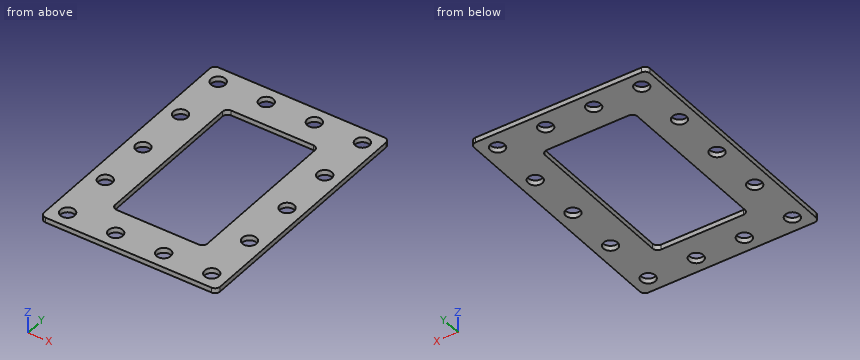
Autodesk Inventor part; units mm, degrees
ref_plane "YZ Plane" through (0, 0, 0) normal (1, 0, 0) x (0, 1, 0)
ref_plane "XZ Plane" through (0, 0, 0) normal (0, 1, 0) x (-1, 0, 0)
ref_plane "XY Plane" through (0, 0, 0) normal (0, 0, 1) x (1, 0, 0)
sketch "Sketch2" plane through (0, 0, 0) normal (0, 0, 1) x (1, 0, 0)
  line L0 (-55, -98) -> (55, -98)
  line L1 (55, -98) -> (55, 98)
  line L2 (55, 98) -> (-55, 98)
  line L3 (-55, 98) -> (-55, -98)
  line L4 (-55, -98) -> (55, 98) construction
  line L5 (55, -98) -> (-55, 98) construction
  line L6 (-105, -148) -> (105, -148)
  line L7 (105, -148) -> (105, 148)
  line L8 (105, 148) -> (-105, 148)
  line L9 (-105, 148) -> (-105, -148)
  point P0 (0, 0)
  dimension "d29" = 110
  dimension "d30" = 196
  dimension "d31" = 50
extrude "Plate2" add sketch "Sketch2" along normal blind 6
sketch "Sketch5" plane through (0, 0, 6) normal (0, 0, 1) x (1, 0, 0)
  line L0 (55, 98) -> (55, -98) construction
  line L1 (55, -98) -> (-55, -98) construction
  line L2 (-55, -98) -> (-55, 98) construction
  line L3 (-55, 98) -> (55, 98) construction
  line L4 (105, -148) -> (-105, -148) construction
  line L5 (105, 148) -> (105, -148) construction
  line L6 (-105, 148) -> (105, 148) construction
  line L7 (-105, -148) -> (-105, 148) construction
  line L8 (-86, 129) -> (86, 129) construction
  line L9 (86, 129) -> (86, -129) construction
  line L10 (86, -129) -> (-86, -129) construction
  line L11 (-86, -129) -> (-86, 129) construction
  line L12 (-55, 0) -> (55, 0) construction
  line L13 (0, 98) -> (0, -98)
  point P0 (0, 0)
  point P1 (0, -129)
  point P2 (-86, 64.5)
  point P3 (-86, 0)
  point P4 (-86, -64.5)
  point P5 (-28.6667, -129)
  point P6 (28.6667, -129)
  point P7 (86, -64.5)
  point P8 (86, 0)
  point P9 (86, 64.5)
  point P10 (28.6667, 129)
  point P11 (-28.6667, 129)
  dimension "d34" = 19
  dimension "d49" = 64.5
  dimension "d50" = 64.5
  dimension "d51" = 57.3333
  dimension "d52" = 57.3333
  dimension "d53" = 57.3333
fillet "Corner Round1" radius 6 8 edges at (-105, -148, 3) (-105, 148, 3) (105, 148, 3) (105, -148, 3) (55, -98, 3) (-55, -98, 3) (-55, 98, 3) (55, 98, 3)
hole "Hole1" at (-86, 129, 6) at (-86, 64.5, 6) at (-86, 0, 6) at (-86, -64.5, 6) at (-86, -129, 6) at (-28.6667, -129, 6) at (28.6667, -129, 6) at (86, -129, 6) at (86, -64.5, 6) at (86, 0, 6) at (86, 64.5, 6) at (86, 129, 6) at (28.6667, 129, 6) at (-28.6667, 129, 6) direction (0, 0, -1) diameter 17 end through all
equation "\"d29\" = ChargingHatch_hight - 2 * Thickness"
equation "\"d30\" = ChargingHatch_width - 2 * Thickness"
equation "\"d59\" = Thickness"
equation "\"d14\" = Thickness"
equation "\"BendReliefWidth\" = Thickness"
equation "\"BendReliefDepth\" = 0.5 * Thickness"
equation "\"CornerReliefSize\" = 4 * Thickness"
equation "\"MinimumRemnant\" = 2 * Thickness"
equation "\"TransitionRadius\" = BendRadius"
equation "\"JacobiRadiusSize\" = BendRadius"
equation "\"GapSize\" = Thickness"
properties part number "PRS 9606 charging flange round_D1200" material "Steel"
Design review of the part built by this model. Coordinates are the model's own, in mm. Coordinates: 2 decimals unless noted, no trailing zeros. Loops run counter-clockwise (first coordinate to the right, second up) from the corner with the lowest first, then second, coordinate; pieces in that order, holes last. Notation, with made-up numbers: M 76,66.25 L 120,66.25 A13 cw 120,73.25 Z; hole C 41.25,3 d8. An arc over 180 degrees is marked long. Use one line per item in the form item = value.
(1) Consider section C-C (y = -64.5). Write out the cut boundary in (x, z).
Return value:
outline = M -105,0 L -94.5,0 L -94.5,6 L -105,6 Z; M -77.5,0 L -55,0 L -55,6 L -77.5,6 Z; M 55,0 L 77.5,0 L 77.5,6 L 55,6 Z; M 94.5,0 L 105,0 L 105,6 L 94.5,6 Z
(2) Consider section A-A (y = 85). Write out the cut boundary in (x, z), and give its area (3 significant figures).
Return value:
outline = M -105,0 L -55,0 L -55,6 L -105,6 Z; M 55,0 L 105,0 L 105,6 L 55,6 Z
area = 600 mm2
(3) Clearance check with flat-ended pins moving along their axes: P1, Ø13.5, axis at x = 86, y = 129, coming from the +Z side; P2, Ø19.5, axis at x = 86, y = -64.5, coming from the -Z side. State where each tip first meets the part, or that it passes through.
Return value:
P1 = through
P2 = 0
(4) Consider section B-B (x = -86). Write out the cut boundary in (y, z), and give its area (3 significant figures).
Return value:
outline = M -148,0 L -137.5,0 L -137.5,6 L -148,6 Z; M -120.5,0 L -73,0 L -73,6 L -120.5,6 Z; M -56,0 L -8.5,0 L -8.5,6 L -56,6 Z; M 8.5,0 L 56,0 L 56,6 L 8.5,6 Z; M 73,0 L 120.5,0 L 120.5,6 L 73,6 Z; M 137.5,0 L 148,0 L 148,6 L 137.5,6 Z
area = 1,270 mm2
(5) For line 1 along X through (y, z) = (129, 3.2); line 2 along Y through (x, z) = (-86, 2.9); line 3 along X through (y, z) = (-64.5, 2), list the stretches that pass through material, from the lowest coordinate up. Write a range as from..to.
Return value:
line_1 = -105..-94.5, -77.5..-37.17, -20.17..20.17, 37.17..77.5, 94.5..105
line_2 = -148..-137.5, -120.5..-73, -56..-8.5, 8.5..56, 73..120.5, 137.5..148
line_3 = -105..-94.5, -77.5..-55, 55..77.5, 94.5..105
(6) Consider section D-D (z = 1.4). Give the number of separate pieces and of enclosed holes in the cut face, and give its area (3 significant figures).
Return value:
separate_pieces = 1
enclosed_holes = 15
area = 37,400 mm2
